from build123d import *

# Parameters (mm, degrees)
F0_W     = 40
F0_H     = 40
F1_DEPTH = 5
F2_R     = 18
F3_DEPTH = 5


with BuildPart() as f1:
    # F0 (on Right) → F1 (new body)
    with BuildSketch(Plane.YZ):
        with Locations((20, 20)):
            Rectangle(F0_W, F0_H)
    extrude(amount=-F1_DEPTH)

    # F2 (on face) → F3 (cut, through all)
    with BuildSketch(Plane.YZ):
        with Locations((20, 20)):
            Circle(F2_R)
    extrude(amount=-F3_DEPTH, mode=Mode.SUBTRACT)


solid = f1.part
Design review of the part built by this model. Coordinates are the model's own, in mm. Coordinates: 2 decimals unless noted, no trailing zeros. Write each loop counter-clockwise with the first axis right and the second up, starting at its lowest first coordinate (ties: lowest second). Pieces come first, ordered by that corner, then holes. Notation, with made-up numbers: (-29, 32.25) - (7, 32.25) arc R29 ccw to (7, 60.25) - close; hole circle Ø3 at (5, 13.5). An arc over 180 degrees is marked (long way). Use one line per item in the form item = value.
Q1. For probe 1 along Z at (x, y) = (-2.75, 20); probe 2 along Y at (x, z) = (-2.5, 31.5); probe 3 along Y at (x, z) = (-1.1, 18.5), list the stretches that pass through material, from the lowest coordinate up.
Taken from the geometry:
probe_1 = 0 to 2, 38 to 40
probe_2 = 0 to 6.15, 33.85 to 40
probe_3 = 0 to 2.06, 37.94 to 40
Q2. Consider section A-A (y = 20). Write out the cut boundary in (x, z).
Taken from the geometry:
outline = (-5, 0) - (0, 0) - (0, 2) - (-5, 2) - close; (-5, 38) - (0, 38) - (0, 40) - (-5, 40) - close
Q3. Consider section C-C (x = -3.55). Write out the cut boundary in (y, z), plus the area to 3 significant figures.
Taken from the geometry:
outline = (0, 0) - (40, 0) - (40, 40) - (0, 40) - close; hole circle Ø36 at (20, 20)
area = 582 mm^2
